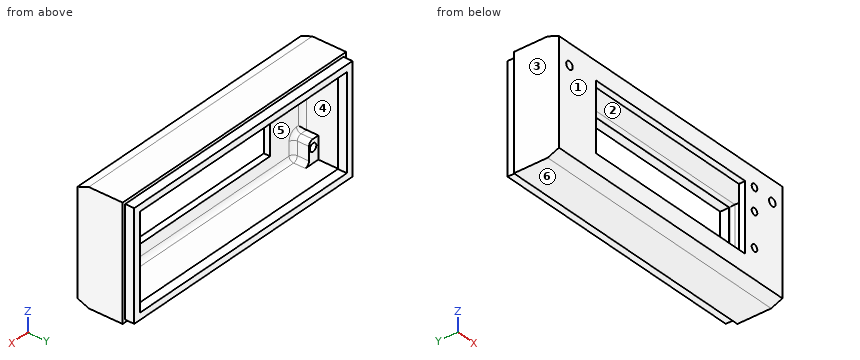
from build123d import *

# Parameters (mm, degrees)
F0_W          = 120
F0_H          = 50
F1_DEPTH      = 10
F1_DEPTH_BACK = 10
F2_T          = -2.8
F3_W          = 80
F3_H          = 30
F4_DEPTH      = 20.001
F6_W          = 5
F6_H          = 10
F7_DEPTH      = 7.2
F8_F1_R       = 2
F8_F2_R       = 2
F9_SIZE2      = 2
F9_SIZE       = 5
F9_2_SIZE2    = 2
F9_2_SIZE     = 5
F10_D         = 3
F12_D         = 3.5
F12_DEPTH     = 5
F12_START     = 5.9405501
F12_TIP       = 1.0515060833
F13_W         = 117.182782799
F13_H         = 47.6424540132
F13_W_2       = 111.182782799
F13_H_2       = 41.6424540132
F14_DEPTH     = 4
F15_R         = 1.2


with BuildPart() as f1:
    # F0 (on Front) → F1 (new body, two sides)
    with BuildSketch(Plane.XZ) as f1_sk:
        Rectangle(F0_W, F0_H)
    extrude(amount=F1_DEPTH)
    extrude(f1_sk.sketch, amount=-F1_DEPTH_BACK)

    # F2
    f2_openings = [f1.faces().sort_by_distance(p)[0] for p in [
        (0, 10, 0),
    ]]
    offset(amount=F2_T, openings=f2_openings)

    # F3 (on face) → F4 (cut, through all)
    with BuildSketch(Plane.XZ.offset(10)):
        Rectangle(F3_W, F3_H)
    extrude(amount=-F4_DEPTH, mode=Mode.SUBTRACT)

    # F6 (on Front) → F7 (join, through all)
    with BuildSketch(Plane.XZ):
        with Locations((54.7, 17.2)):
            Rectangle(F6_W, F6_H)
        with Locations((54.7, -17.2)):
            Rectangle(F6_W, F6_H)
        with Locations((-54.7, 17.2)):
            Rectangle(F6_W, F6_H)
        with Locations((-54.7, -17.2)):
            Rectangle(F6_W, F6_H)
    extrude(amount=F7_DEPTH)

    # F8: fillet of radius 2 on 14 edges, made by hand

    # F8_f1
    f8_f1_edges = [f1.edges().sort_by_distance(p)[0] for p in [
        (52.2, -3.6, 12.2),
        (-52.2, -3.6, 12.2),
        (-52.2, -3.6, -12.2),
        (52.2, -3.6, -12.2),
    ]]
    fillet(f8_f1_edges, radius=F8_F1_R)

    # F8_f2
    f8_f2_edges = [f1.edges().sort_by_distance(p)[0] for p in [
        (52.2, -7.2, -18.2),
        (52.2, -7.2, 18.2),
        (0, -7.2, 22.2),
        (-52.2, -7.2, 18.2),
        (-52.2, -3.6, 22.2),
        (-57.2, -3.6, 12.2),
        (-57.2, -7.2, 0),
        (0, -7.2, -22.2),
        (-52.2, -7.2, -18.2),
        (-52.2, -3.6, -22.2),
        (-52.7857864376, -7.2, -12.7857864376),
        (-52.7857864376, -7.2, 12.7857864376),
        (52.7857864376, -7.2, 12.7857864376),
        (52.7857864376, -7.2, -12.7857864376),
    ]]
    fillet(f8_f2_edges, radius=F8_F2_R)

    # F9
    f9_edges = [f1.edges().sort_by_distance(p)[0] for p in [
        (0, -10, -25),
    ]]
    f9_side = f1.faces().sort_by_distance((0, 0, -25))[0]
    chamfer(f9_edges, length=F9_SIZE, length2=F9_SIZE2, reference=f9_side)

    # F9#2
    f9_2_edges = [f1.edges().sort_by_distance(p)[0] for p in [
        (0, -10, 25),
    ]]
    f9_2_side = f1.faces().sort_by_distance((0, 0, 25))[0]
    chamfer(f9_2_edges, length=F9_2_SIZE, length2=F9_2_SIZE2, reference=f9_2_side)

    # F10 (through all)
    with Locations(Plane.XZ.offset(10)):
        with Locations((45, 5), (45, 15), (45, -10)):
            Hole(F10_D / 2)

    # F12
    # its depths count from where the whole tool has entered the part; down to there all is cleared
    with Locations(Plane(origin=(0, 0, 0), x_dir=(1, 0, 0), z_dir=(0, 1, 0))):
        with Locations((54.5504838228, -13.8078443706), (-54.356444627, -13.8078443706)):
            Hole(F12_D / 2, depth=F12_START)
    with Locations(Plane(origin=(0, 0, 0), x_dir=(1, 0, 0), z_dir=(0, 1, 0))):
        with Locations((54.5504838228, -13.8078443706, -F12_START), (-54.356444627, -13.8078443706, -F12_START), (-54.356444627, 15.7220419496, 0), (54.5504838228, 15.7220419496, 0)):
            Hole(F12_D / 2, depth=F12_DEPTH)
            with Locations((0, 0, -(F12_DEPTH + F12_TIP / 2))):  # 118° drill point
                Cone(0, F12_D / 2, F12_TIP, mode=Mode.SUBTRACT)

    # F13 (on face) → F14 (join)
    with BuildSketch(Plane(origin=(0, 10, 0), x_dir=(-1, 0, 0), z_dir=(0, 1, 0))):
        with Locations((-0.0398587435, -0.1178945079)):
            Rectangle(F13_W, F13_H)
        with Locations((-0.0398587435, -0.1178945079)):
            Rectangle(F13_W_2, F13_H_2, mode=Mode.SUBTRACT)
    extrude(amount=F14_DEPTH)

    # F15
    f15_edges = [f1.edges().sort_by_distance(p)[0] for p in [
        (0, 10, 22.2),
        (-57.2, 10, 0),
        (0, 10, -22.2),
        (57.2, 10, 0),
    ]]
    fillet(f15_edges, radius=F15_R)


solid = f1.part
Source: CAD feature listing. Evaluate the final solid. Frame: model axes, mm. Face numbers are marked on the shaded views. A direction names the side the tool comes from. Coordinates: 2 decimals unless noted, no trailing zeros. Write each loop counter-clockwise with the first axis right and the second up, starting at its lowest first coordinate (ties: lowest second). Pieces come first, ordered by that corner, then holes. Notation, with made-up numbers: M -17,-14 L 30,-14 A14 ccw 30,0 Z; hole C -13.5,-34 d6. An arc over 180 degrees is marked long. Use a Markdown table: item, result.
1) Reachability of the marked faces 1 and 2 from +Z, -Z, +X, -X, +Y, -Y: full face, straight path, thin tool, end or side. Return the list, or none.
Conclusion:
| item | result |
|---|---|
| face 1 | +Z, -Z, +X, -X, -Y |
| face 2 | none |
2) Section C-C, the plane y = 1.5. Output: boundary loops of the cut face in (x, z), then the cut area to 3 significant figures.
Conclusion:
| item | result |
|---|---|
| outline | M -60,-25 L 60,-25 L 60,25 L -60,25 Z; hole M -57.2,-22.2 L 57.2,-22.2 L 57.2,22.2 L -57.2,22.2 Z |
| area | 921 mm^2 |
3) Section B-B, the plane z = 5. Output: boundary loops of the cut face in (x, y), then the cut area to 3 significant figures.
Conclusion:
| item | result |
|---|---|
| outline | M -60,-10 L -40,-10 L -40,-7.2 L -55.2,-7.2 A2 cw -57.2,-5.2 L -57.2,8.8 A1.2 cw -56,10 L -55.55,10 L -55.55,14 L -58.55,14 L -58.55,10 L -60,10 Z; M 40,-10 L 43.5,-10 L 43.5,-7.2 L 40,-7.2 Z; M 46.5,-10 L 60,-10 L 60,10 L 58.63,10 L 58.63,14 L 55.63,14 L 55.63,10 L 56,10 A1.2 cw 57.2,8.8 L 57.2,-7.2 L 46.5,-7.2 Z |
| area | 225 mm^2 |
4) First-contact query: pin 1 Ø10 at (x, z) = (41, -8) entering from +Y; pin 2 Ø2 at (x, y) = (-10, 12.5) entering from +Z; pin 3 Ø3.5 at (x, z) = (-52.5, -15) entering from +Y; pin 4 Ø8 at (x, z) = (18, 9) entering from -Y. Flat tips, straight axial feed; report the tip coordinate or a pass-through.
Conclusion:
| item | result |
|---|---|
| pin 1 | stops at y = -7.2 |
| pin 2 | stops at z = 23.7 |
| pin 3 | stops at y = 0 |
| pin 4 | passes through |
5) Section A-A, the plane x = 45. Give the number of separate pieces and of enclosed holes in the cut face, then the cut area to 3 significant figures.
Conclusion:
| item | result |
|---|---|
| separate pieces | 4 |
| enclosed holes | 0 |
| area | 227 mm^2 |
6) Section D-D, the plane x = 9. Output: boundary loops of the cut face in (y, z), then the cut area to 3 significant figures.
Conclusion:
| item | result |
|---|---|
| outline | M -10,-23 L -5,-25 L 10,-25 L 10,-23.94 L 14,-23.94 L 14,-20.94 L 10,-20.94 L 10,-21 A1.2 cw 8.8,-22.2 L -5.2,-22.2 A2 cw -7.2,-20.2 L -7.2,-15 L -10,-15 Z; M -10,15 L -7.2,15 L -7.2,20.2 A2 cw -5.2,22.2 L 8.8,22.2 A1.2 cw 10,21 L 10,20.7 L 14,20.7 L 14,23.7 L 10,23.7 L 10,25 L -5,25 L -10,23 Z |
| area | 169 mm^2 |
7) Ray query, L1, parallel to Z at x = -36, y = -3.25; L2, parallel to X at y = -2, z = -9.5; L3, parallel to Z at x = 45, y = -8.95. Return the intervals inside material, ascending.
Conclusion:
| item | result |
|---|---|
| L1 | z = -25 to -22.2, 22.2 to 25 |
| L2 | x = -60 to -57.2, 57.2 to 60 |
| L3 | z = -23.42 to -11.5, -8.5 to 3.5, 6.5 to 13.5, 16.5 to 23.42 |
8) Mould query, pull axis X, two halves, no side actions, for the marked faces 3, 4, 5 and 6. Classes: pulls with the +X half, pulls with the -X half, needs draft (parallel to the pull), parting line crosses it, or undercut.
Conclusion:
| item | result |
|---|---|
| face 3 | pulls with the -X half |
| face 4 | undercut |
| face 5 | undercut |
| face 6 | needs draft |
